from build123d import *

# Parameters (mm, degrees)
SKETCH_2_R             = 8
SKETCH_2_R_2           = 10
SM_BASE_FLANGE_1_DEPTH = 4


# Sheet-metal steps are written as plain solids
with BuildPart() as part:
    # Sketch 2 → Базовая кромка1 (new body)
    with BuildSketch(Plane.XY):
        with BuildLine():
            Line((-160.225, 17.998593695), (-0.25, 19.998437439))
            ThreePointArc((-0.25, 19.998437439), (20, 0), (-0.25, -19.998437439))
            Line((-0.25, -19.998437439), (-160.225, -17.998593695))
            ThreePointArc((-160.225, -17.998593695), (-178, 0), (-160.225, 17.998593695))
        make_face()
        with Locations((-160, 0)):
            Circle(SKETCH_2_R, mode=Mode.SUBTRACT)
        Circle(SKETCH_2_R_2, mode=Mode.SUBTRACT)
    extrude(amount=-SM_BASE_FLANGE_1_DEPTH)


solid = part.part
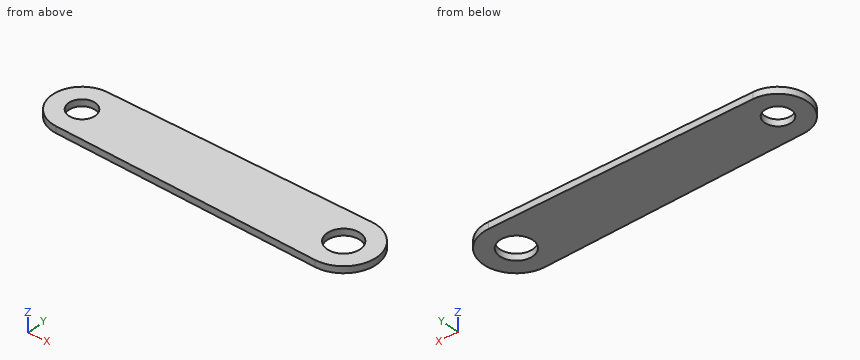
Model file for the job. Use its own axes, mm. Give positions to 0.01 mm unless a question says otherwise; leave off trailing zeros. Order: outer loops, then holes, each group sorted by start corner. A loop starts at its lowest first (then second) coordinate and runs counter-clockwise, first axis right, second up. Notation, with made-up numbers: M -19.5,13.25 L -6.5,13.25 A8 ccw -6.5,17.25 Z; hole C 50.25,-5 d3. An arc over 180 degrees is marked long. Write item = value, one per line.
Q1. Cut at A-A, the plane x = -3. List the corners of the cut face in (y, z).
Derived:
outline = M -19.96,-4 L -9.54,-4 L -9.54,0 L -19.96,0 Z; M 9.54,-4 L 19.96,-4 L 19.96,0 L 9.54,0 Z
Q2. Cut at C-C, the plane z = -1.9. List the corners of the cut face in (x, y) (3 decimals).
Derived:
outline = M -160.225,-17.999 L -0.25,-19.998 A20 ccw long -0.25,19.998 L -160.225,17.999 A18 ccw Z; hole C -160,0 d16; hole C 0,0 d20
Q3. Cut at B-B, the plane y = 2. List the corners of the cut face in (x, z).
Derived:
outline = M -177.89,-4 L -167.75,-4 L -167.75,0 L -177.89,0 Z; M -152.25,-4 L -9.8,-4 L -9.8,0 L -152.25,0 Z; M 9.8,-4 L 19.9,-4 L 19.9,0 L 9.8,0 Z
Q4. Flat gauge pins, fed straight in: pin 1 (2 mm diameter, centred on y = -12, z = -2.5, fed in from +X); pin 2 (16 mm diameter, centred on x = 0, y = 0, fed in from +Z). Where does each tip first touch, or does it go through?
Derived:
pin_1 = 16.7
pin_2 = through
Q5. Cut at D-D, the plane x = -129.5. List the corners of the cut face in (y, z).
Derived:
outline = M -18.38,-4 L 18.38,-4 L 18.38,0 L -18.38,0 Z
Q6. Drill centre lines: line 1 (Y direction, x = 0, z = -2.8); line 2 (X direction, y = -3, z = -2.95); line 3 (Y direction, x = -160, z = -2.1). Where is each one in solid material? Low to high. Write a range as [from, to].
Derived:
line_1 = [-20, -10], [10, 20]
line_2 = [-177.75, -167.42], [-152.58, -9.54], [9.54, 19.77]
line_3 = [-18, -8], [8, 18]
